Read the model definition and answer for the solid it produces. Units are mm, in the model's axes. Face numbers are marked on the shaded views. A direction names the side the tool comes from. Round coordinates to 2 decimals unless told otherwise and drop trailing zeros. Order: outer loops, then holes, each group sorted by start corner. A loop starts at its lowest first (then second) coordinate and runs counter-clockwise, first axis right, second up. Notation, with made-up numbers: M -22.75,-20 L -12.75,-20 A32 ccw -12.75,16 Z; hole C 56,-36.75 d1. An arc over 180 degrees is marked long. Answer as CSV lines item,"result".
Autodesk Inventor part; units mm, degrees
ref_plane "YZ Plane" through (0, 0, 0) normal (1, 0, 0) x (0, 1, 0)
ref_plane "XZ Plane" through (0, 0, 0) normal (0, 1, 0) x (-1, 0, 0)
ref_plane "XY Plane" through (0, 0, 0) normal (0, 0, 1) x (1, 0, 0)
sketch "Sketch1" plane through (0, 0, 0) normal (0, 0, 1) x (1, 0, 0)
  circle A0 centre (0, 0) radius 25.5
  dimension "d0" = 51
extrude "Extrusion1" add sketch "Sketch1" along normal blind 3
sketch "Sketch2" plane through (0, 0, 3) normal (0, 0, 1) x (1, 0, 0)
  circle A0 centre (0, 0) radius 25.5
  circle A1 centre (0, 0) radius 14.5
  dimension "d3" = 29
extrude "Extrusion2" add sketch "Sketch2" along normal blind 2 contours A1
sketch "Sketch3" plane through (0, 0, 0) normal (0, 0, -1) x (-1, 0, 0)
  circle A0 centre (0, 0) radius 25.5
  circle A1 centre (0, 0) radius 8
  dimension "d6" = 16
extrude "Extrusion3" add sketch "Sketch3" along normal blind 9.5 contours A1
sketch "Sketch4" plane through (0, 0, 5) normal (0, 0, 1) x (1, 0, 0)
  circle A0 centre (0, 0) radius 14.5
  circle A1 centre (0, 0) radius 3
  dimension "d9" = 6
extrude "Extrusion4" cut sketch "Sketch4" against normal through all contours A1
sketch "Sketch5" plane through (0, 0, 3) normal (0, 0, 1) x (1, 0, 0)
  circle A0 centre (0, 0) radius 25.5
  circle A1 centre (0, 0) radius 20.5
  circle A2 centre (0, 20.5) radius 1.5
  circle A3 centre (-14.4957, 14.4957) radius 1.5
  circle A4 centre (-20.5, 0) radius 1.5
  circle A5 centre (-14.4957, -14.4957) radius 1.5
  circle A6 centre (0, -20.5) radius 1.5
  circle A7 centre (14.4957, -14.4957) radius 1.5
  circle A8 centre (20.5, 0) radius 1.5
  circle A9 centre (14.4957, 14.4957) radius 1.5
  dimension "d12" = 41
  dimension "d13" = 3
  dimension "d16" = 360
extrude "Extrusion5" cut sketch "Sketch5" against normal through all contours A1 A8 | A1 A8 | A9 A1 | A1 A9 | A7 A1 | A1 A7 | A2 A1 | A1 A2 | A6 A1 | A1 A6 | A3 A1 | A1 A3 | A5 A1 | A1 A5 | A4 A1 | A1 A4
sketch "Sketch6" plane through (0, 0, -9.5) normal (0, 0, -1) x (-1, 0, 0)
  circle A0 centre (0, 0) radius 3
hole "Hole1" at (0, 0, -9.5) direction (0, 0, 1) diameter 8.9175 depth 13 counterbore diameter 9 counterbore depth 10
properties part number "08 CYLINDER REAR COVER" material "Steel AISI 1020 107 HR"
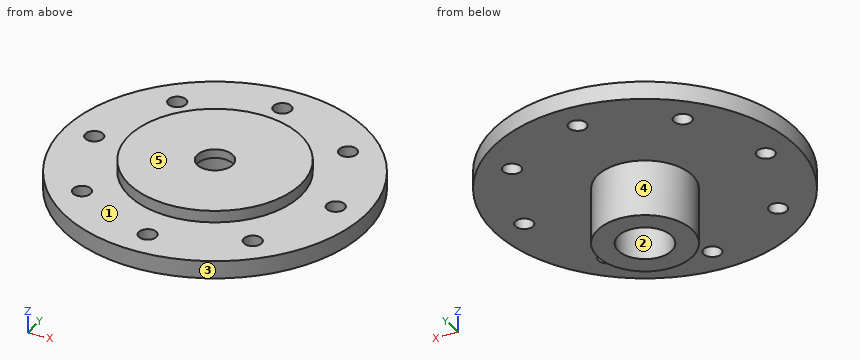
Item 1: A cutting plane is placed at C-C, the plane z = -2.5. Determine the outline of the cut face in (x, y).
Ans:
outline,"C 0,0 d16; hole C 0,0 d9"
Item 2: Determine the mould class of the marked faces 1, 2 and 3 for opening direction X: +X half, -X half, draft (parallel to the pull), parting line (faces both ways), or undercut.
Ans:
face 1,"draft"
face 2,"undercut"
face 3,"parting line"
Item 3: A cutting plane is placed at D-D, the plane y = 20.5. Determine the outline of the cut face in (x, z).
Ans:
outline,"M -15.17,0 L -1.5,0 L -1.5,3 L -15.17,3 Z; M 1.5,0 L 15.17,0 L 15.17,3 L 1.5,3 Z"
Item 4: Find the intervals of material crossed by probe 1 along Y at (x, z) = (0, 2.3); probe 2 along Z at (x, y) = (3.5, 20); probe 3 along Y at (x, z) = (-1, -2), in increasing order. Write a range as [from, to].
Ans:
probe 1,"[-25.5, -22], [-19, -4.46], [4.46, 19], [22, 25.5]"
probe 2,"[0, 3]"
probe 3,"[-7.94, -4.39], [4.39, 7.94]"
Item 5: Flat-ended cylindrical pins translate along their axes: pin 1 (5 mm diameter, centred on x = 20.5, y = 0, fed in from -Z); pin 2 (3 mm diameter, centred on y = -19.5, z = 0.5, fed in from +X); pin 3 (2.5 mm diameter, centred on x = 14.5, y = 14.5, fed in from -Z); pin 4 (4 mm diameter, centred on y = -9, z = -3.5, fed in from +X). Find the tip coordinate at first contact, or state that the pin passes through.
Ans:
pin 1,"z = 0"
pin 2,"x = 18.06"
pin 3,"through"
pin 4,"x = 3.87"
Item 6: A cutting plane is placed at A-A, the plane y = 0. Give the number of separate pieces and of enclosed holes in the cut face, and give its area (3 significant figures).
Ans:
separate pieces,"4"
enclosed holes,"0"
area,"219 mm2"
Item 7: A tool of negligible diameter and unlimited length cuts with its end or side. For the marked faces 4 and 5, from which of +Z, -Z, +X, -X, +Y, -Y can it reach the whole face along a straight path? Write none if from no direction.
Ans:
face 4,"-Z"
face 5,"+Z, +X, -X, +Y, -Y"
